```python
from build123d import *

# Parameters (mm, degrees)
SKETCH_R        = 25
PAD_DEPTH       = 11
SKETCH001_W     = 10
SKETCH001_H     = 32
PAD001_DEPTH    = 11
SKETCH002_R     = 10
PAD002_DEPTH    = 11
SKETCH003_R     = 7
POCKET_DEPTH    = 8
SKETCH004_R     = 2.25
POCKET001_DEPTH = 11
POCKET002_DEPTH = 8
SKETCH006_R     = 2
POCKET003_DEPTH = 10


with BuildPart() as part:
    # Sketch → Pad (new body)
    with BuildSketch(Plane.XY):
        Circle(SKETCH_R)
    extrude(amount=PAD_DEPTH)

    # Sketch001 → Pad001 (new body)
    with BuildSketch(Plane.XY.offset(11)):
        Rectangle(SKETCH001_W, SKETCH001_H)
    extrude(amount=PAD001_DEPTH)

    # Sketch002 → Pad002 (new body)
    with BuildSketch(Plane.XY.offset(11)):
        Circle(SKETCH002_R)
    extrude(amount=PAD002_DEPTH)

    # Sketch003 → Pocket (cut)
    with BuildSketch(Plane.XY.offset(22)):
        Circle(SKETCH003_R)
    extrude(amount=-POCKET_DEPTH, mode=Mode.SUBTRACT)

    # Sketch004 → Pocket001 (cut)
    with BuildSketch(Plane(origin=(0, 0, 0), x_dir=(1, 0, 0), z_dir=(0, 0, -1))):
        with Locations((-10, 17.320508)):
            Circle(SKETCH004_R)
        with Locations((20, 0)):
            Circle(SKETCH004_R)
        with Locations((-10, -17.320508)):
            Circle(SKETCH004_R)
    extrude(amount=-POCKET001_DEPTH, mode=Mode.SUBTRACT)

    # Sketch005 → Pocket002 (cut)
    with BuildSketch(Plane(origin=(0, 0, 0), x_dir=(1, 0, 0), z_dir=(0, 0, -1))):
        with BuildLine():
            ThreePointArc((-2.995739, 5.15983), (-4.223459, 4.214344), (-5.16629, 2.984585))
            ThreePointArc((-5.16629, 2.984585), (-7.987609, -0.004867), (-5.153374, -2.982076))
            ThreePointArc((-5.153374, -2.982076), (-4.202268, -4.217936), (-2.962876, -5.164437))
            ThreePointArc((-2.962876, -5.164437), (0.02321, -7.983708), (2.996215, -5.150646))
            ThreePointArc((2.996215, -5.150646), (4.257192, -4.171102), (5.217582, -2.895476))
            ThreePointArc((5.217582, -2.895476), (7.999941, 0.115474), (5.179963, 3.09122))
            ThreePointArc((5.179963, 3.09122), (4.223984, 4.306463), (2.990483, 5.238766))
            ThreePointArc((2.990483, 5.238766), (-0.039555, 7.999739), (-2.995739, 5.15983))
        make_face()
    extrude(amount=-POCKET002_DEPTH, mode=Mode.SUBTRACT)

    # Sketch006 → Pocket003 (cut)
    with BuildSketch(Plane(origin=(-5, 0, 0), x_dir=(0, -1, 0), z_dir=(-1, 0, 0))):
        with Locations((-12, 18)):
            Circle(SKETCH006_R)
        with Locations((12, 18)):
            Circle(SKETCH006_R)
    extrude(amount=-POCKET003_DEPTH, mode=Mode.SUBTRACT)


solid = part.part
```
Build history of the part. All positions in model axes, mm. A direction names the side the tool comes from. Round coordinates to 2 decimals unless told otherwise and drop trailing zeros. Order: outer loops, then holes, each group sorted by start corner. A loop starts at its lowest first (then second) coordinate and runs counter-clockwise, first axis right, second up. Notation, with made-up numbers: (-25.5, 9.25) - (18.5, 9.25) arc R11 ccw to (18.5, 20.25) - close; hole circle Ø10 at (28, 24.25). An arc over 180 degrees is marked (long way). Use a Markdown table: item, result.
1) Saw through at A-A on y = -12. Write the cut outline in (x, z).
Recorded:
| item | result |
|---|---|
| outline | (-21.93, 0) - (21.93, 0) - (21.93, 11) - (5, 11) - (5, 16) - (-5, 16) - (-5, 11) - (-21.93, 11) - close; (-5, 20) - (5, 20) - (5, 22) - (-5, 22) - close |
2) Saw through at D-D on x = -11. Write the cut outline in (y, z).
Recorded:
| item | result |
|---|---|
| outline | (-22.45, 0) - (-19.34, 0) - (-19.34, 11) - (-22.45, 11) - close; (-15.3, 0) - (15.3, 0) - (15.3, 11) - (-15.3, 11) - close; (19.34, 0) - (22.45, 0) - (22.45, 11) - (19.34, 11) - close |
3) Saw through at C-C on z = 6.25. Write the cut outline in (x, y), and give its area (3 significant figures).
Recorded:
| item | result |
|---|---|
| outline | circle Ø50 at (0, 0); hole circle Ø4.5 at (-10, -17.32); hole circle Ø4.5 at (-10, 17.32); hole (-5.17, -2.98) arc R5.97 ccw to (-3, -5.16) arc R3 ccw to (2.99, -5.24) arc R6.03 ccw to (5.18, -3.09) arc R3 ccw to (5.22, 2.9) arc R6.04 ccw to (3, 5.15) arc R2.98 ccw to (-2.96, 5.16) arc R5.95 ccw to (-5.15, 2.98) arc R2.99 ccw to start; hole circle Ø4.5 at (20, 0) |
| area | 1,760 mm² |
4) Wall check: L1, parallel to Y at x = -10, z = 6.75; L2, parallel to Y at x = -1.5, z = 19; L3, parallel to X at y = 14.5, z = 19. Give the ranges that are in metal, low to high.
Recorded:
| item | result |
|---|---|
| L1 | y = -22.91 to -19.57, -15.07 to 15.07, 19.57 to 22.91 |
| L2 | y = -16 to -13.73, -10.27 to -6.84, 6.84 to 10.27, 13.73 to 16 |
| L3 | x = -5 to 5 |
5) Saw through at B-B on z = 13.25. Write the cut outline in (x, y), and give its area (3 significant figures).
Recorded:
| item | result |
|---|---|
| outline | (-5, -16) - (5, -16) - (5, -8.66) arc R10 ccw to (5, 8.66) - (5, 16) - (-5, 16) - (-5, 8.66) arc R10 ccw to (-5, -8.66) - close |
| area | 443 mm² |
6) Flat gauge pins, fed straight in: pin 1 Ø1 at (x, y) = (12, 4) entering from -Z; pin 2 Ø6 at (x, y) = (-19.5, -2) entering from +Z; pin 3 Ø2 at (y, z) = (-12, 18) entering from -X; pin 4 Ø4 at (x, y) = (2, 0) entering from +Z. Where does each tip first touch, or does it go through?
Recorded:
| item | result |
|---|---|
| pin 1 | stops at z = 0 |
| pin 2 | stops at z = 11 |
| pin 3 | passes through |
| pin 4 | stops at z = 14 |
7) Pull direction X, two halves, no side cores. Call faces 6 (the face through (8, 0, 4)), 7 (the face through (0, -12, 20)), 8 (the face through (5, 12, 15)), 9 (the face through (-0.04, 7.983, 3.944)): pulls with the +X half, pulls with the -X half, needs draft (parallel to the pull), parting line crosses it, or undercut.
Recorded:
| item | result |
|---|---|
| face 6 | undercut |
| face 7 | needs draft |
| face 8 | pulls with the +X half |
| face 9 | undercut |
8) Tool access for faces 1 (the face through (-4.22, 4.2, 3.94)), 2 (the face through (10, 0, 16)), 3 (the face through (5, -12, 15)), 4 (the face through (22.146, -0.676, 5.423)), 5 (the face through (-0.1, 7.3, 22)): list every direction of +Z, -Z, +X, -X, +Y, -Y with a clear straight run to the whole face (end or side of a thin tool).
Recorded:
| item | result |
|---|---|
| face 1 | -Z |
| face 2 | +Z, +X |
| face 3 | +Z, +X, -Y |
| face 4 | +Z, -Z |
| face 5 | +Z, +X, -X, +Y, -Y |
